The listing builds one solid part. Answer for the finished solid, in the listing's coordinates (mm). A direction names the side the tool comes from. Give positions to 0.01 mm unless a question says otherwise; leave off trailing zeros. Write each loop counter-clockwise with the first axis right and the second up, starting at its lowest first coordinate (ties: lowest second). Pieces come first, ordered by that corner, then holes. Notation, with made-up numbers: (-37.5, -39) - (-4.5, -39) arc R8 cw to (-4.5, -29) - close; hole circle Ø5 at (-19.75, -6). An arc over 180 degrees is marked (long way). Answer in a Markdown table with one row per item. Add a question column.
from build123d import *

# Parameters (mm, degrees)
SKETCH1_W           = 254
SKETCH1_H           = 101.6
BOSS_EXTRUDE1_DEPTH = 6.35
SKETCH5_W           = 254
SKETCH5_H           = 101.6
SKETCH5_W_2         = 241.3
SKETCH5_H_2         = 88.9
BOSS_EXTRUDE4_DEPTH = 101.6
SKETCH6_W           = 254
SKETCH6_H           = 101.6
BOSS_EXTRUDE5_DEPTH = 6.35


with BuildPart() as part:
    # Sketch1 → Boss-Extrude1 (new body)
    with BuildSketch(Plane(origin=(0, 0, 0), x_dir=(1, 0, 0), z_dir=(0, 1, 0))):
        Rectangle(SKETCH1_W, SKETCH1_H)
    extrude(amount=BOSS_EXTRUDE1_DEPTH)

    # Sketch5 → Boss-Extrude4 (add)
    with BuildSketch(Plane(origin=(0, 6.35, 0), x_dir=(1, 0, 0), z_dir=(0, 1, 0))):
        Rectangle(SKETCH5_W, SKETCH5_H)
        Rectangle(SKETCH5_W_2, SKETCH5_H_2, mode=Mode.SUBTRACT)
    extrude(amount=BOSS_EXTRUDE4_DEPTH)

    # Sketch6 → Boss-Extrude5 (add)
    with BuildSketch(Plane(origin=(0, 107.95, 0), x_dir=(1, 0, 0), z_dir=(0, 1, 0))):
        Rectangle(SKETCH6_W, SKETCH6_H)
    extrude(amount=BOSS_EXTRUDE5_DEPTH)


solid = part.part
1. A tool of negligible diameter and unlimited length cuts with its end or side. For faces 1 (the face through (-2, 6.35, -1)), 2 (the face through (-127, 56, 1)), from which of +Z, -Z, +X, -X, +Y, -Y can it reach the whole face along a straight path? Write none if from no direction.
2. Straight lines are drawn through the part: L1, parallel to Z at x = -106, y = 46; L2, parallel to Y at x = -63, z = -9; L3, parallel to X at y = 93, z = 18. For each, find the intervals that lie inside material, in ascending order. Write a range as [from, to].
3. The mould has two halves that part along Y. Classify faces 3 (the face through (-2, 107.95, -1)), 4 (the face through (-2, 56, 50.8)), 5 (the face through (-2, 0, -1)): +Y half, -Y half, draft (parallel to the pull), parting line (faces both ways), or undercut.
4. Section A-A (y = 20) is taken. Give the vertices of the cut face in (x, z).
5. Section B-B (x = 50.5) is taken. Give the vertices of the cut face in (y, z).
Geometry check:
| question | item | result |
|---|---|---|
| 1 | face 1 | none |
| 1 | face 2 | +Z, -Z, -X, +Y, -Y |
| 2 | L1 | [-50.8, -44.45], [44.45, 50.8] |
| 2 | L2 | [0, 6.35], [107.95, 114.3] |
| 2 | L3 | [-127, -120.65], [120.65, 127] |
| 3 | face 3 | undercut |
| 3 | face 4 | draft |
| 3 | face 5 | -Y half |
| 4 | outline | (-127, -50.8) - (127, -50.8) - (127, 50.8) - (-127, 50.8) - close; hole (-120.65, -44.45) - (120.65, -44.45) - (120.65, 44.45) - (-120.65, 44.45) - close |
| 5 | outline | (0, -50.8) - (114.3, -50.8) - (114.3, 50.8) - (0, 50.8) - close; hole (6.35, -44.45) - (107.95, -44.45) - (107.95, 44.45) - (6.35, 44.45) - close |
